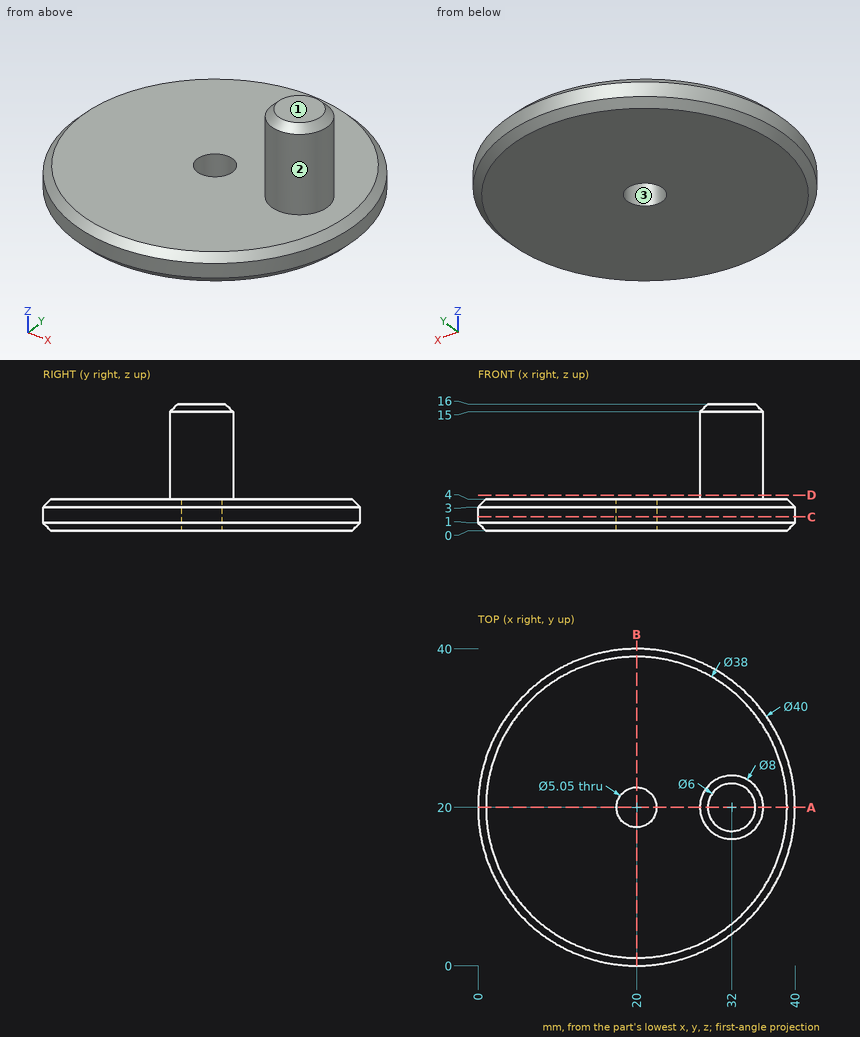
Can you work these out from the drawing? Everything is in mm from the part's minimum corner. Round coordinates to 2 decimals unless told otherwise and drop trailing zeros. Loops run counter-clockwise (first coordinate to the right, second up) from the corner with the lowest first, then second, coordinate; pieces in that order, holes last.
1. We'd pull the mould along X, two halves only. Please class the marked faces 1, 2 and 3: +X half, -X half, draft (parallel to the pull), parting line (faces both ways), or undercut.
Answer list:
face 1: draft
face 2: parting line
face 3: undercut
2. If I drill on line 1 along Y through (x, z) = (20, 2.6) (3 decimals); line 2 along Z through (x, y) = (31.5, 15); line 3 along Y through (x, z) = (30, 11.5), over which ranges is the centre line in solid material (lowest first)?
Answer list:
line 1: y = 0 to 17.475, 22.525 to 40
line 2: z = 0 to 4
line 3: y = 16.54 to 23.46
3. If we section it at C-C on z = 1.75: Write out the boundary of the cut face in (x, y) (3 decimals).
Answer list:
outline: circle Ø40 at (20, 20); hole circle Ø5.05 at (20, 20)
4. For P1, Ø6, axis at x = 34, y = 31, coming from the +Z side; P2, Ø6, axis at y = 14, z = 11.5, coming from the +X side; P3, Ø8, axis at y = 24, z = 5, coming from the +X side, each with a flat end and sliding along its axis, tell me the tip position at first contact or that it passes through.
Answer list:
P1: stops at z = 4
P2: stops at x = 34.65
P3: stops at x = 39.99
5. If we section it at D-D on z = 4.5: Write out the boundary of the cut face in (x, y).
Answer list:
outline: circle Ø8 at (32, 20)
6. If we section it at B-B on x = 20: Write out the boundary of the cut face in (y, z) (3 decimals).
Answer list:
outline: (0, 1) - (1, 0) - (17.475, 0) - (17.475, 4) - (1, 4) - (0, 3) - close; (22.525, 0) - (39, 0) - (40, 1) - (40, 3) - (39, 4) - (22.525, 4) - close
7. If we section it at A-A on y = 20: Write out the boundary of the cut face in (x, z) (3 decimals), plus the area to 3 significant figures.
Answer list:
outline: (0, 1) - (1, 0) - (17.475, 0) - (17.475, 4) - (1, 4) - (0, 3) - close; (22.525, 0) - (39, 0) - (40, 1) - (40, 3) - (39, 4) - (36, 4) - (36, 15) - (35, 16) - (29, 16) - (28, 15) - (28, 4) - (22.525, 4) - close
area: 233 mm2
